Geometry: final body of the model. Coordinates: model frame, mm. Face numbers are marked on the shaded views. A direction names the side the tool comes from. Give positions to 0.01 mm unless a question says otherwise; leave off trailing zeros. Write each loop counter-clockwise with the first axis right and the second up, starting at its lowest first coordinate (ties: lowest second). Pieces come first, ordered by that corner, then holes. Notation, with made-up numbers: (42, 42) -> (50, 42) arc R23 ccw to (50, 54) -> close; hole circle Ø2 at (60, 22.25). An arc over 180 degrees is marked (long way). Answer as a JSON object with one key per item and string values.
from build123d import *

# Parameters (mm, degrees)
F2_R     = 6.2211982037
F3_DEPTH = 19.1516
F4_DEPTH = 55.372
F5_SIZE  = 3.302


# Not quite as in the source:
# - the program builds the solid bodies; features that only make, move or delete a surface that nothing else refers to are left out


with BuildPart() as f1:
    # F0 (on Top) → F1 (revolve)
    with BuildSketch(Plane.XY):
        Polygon((-17.0599853833, 6.2996733477), (-20.4250291926, 4.9693077386), (-13.2254017106, -8.4908647026), (-8.2169655835, -3.2476578449), (-3.9128408491, -8.4126079255), (3.521556964, 4.8910505621), (-2.2694479322, 4.8910505621), (-5.1649496812, 0), (-8.2952223605, 2.6998602059), (-12.2546622766, -1.8907947353), align=None)
    revolve(axis=Axis((-9.930120464, 11.8798027962, 0), (1, 0, 0)))

    # F2 (on Right) → F3 (join)
    with BuildSketch(Plane.YZ):
        with Locations((11.7291258648, 0)):
            Circle(F2_R)
    extrude(amount=-F3_DEPTH)

    # F4 (add): a face of the model
    f4_faces = [f1.faces().sort_by_distance(p)[0] for p in [
        (0, 11.7291258648, 0),
    ]]
    extrude(f4_faces, amount=F4_DEPTH)

    # F5
    f5_edges = [f1.edges().sort_by_distance(p)[0] for p in [
        (55.372, 5.507928, 0),
    ]]
    chamfer(f5_edges, length=F5_SIZE)


solid = f1.part
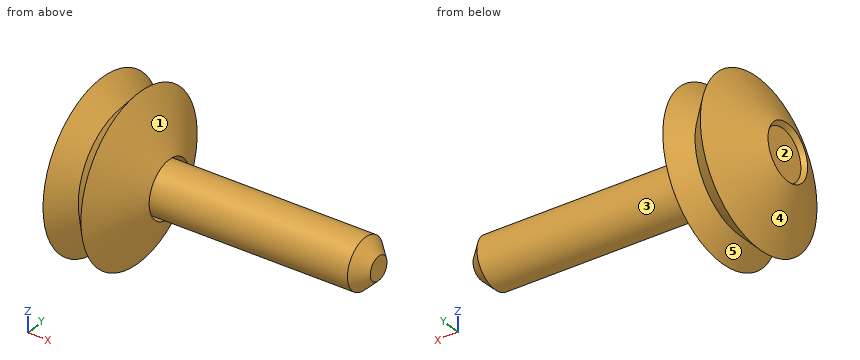
Q1. Set-up query: the marked faces 3, 4 and 5. Return all of +Z, -Z, +X, -X, +Y, -Y with unobstructed straight access to the full face (end or side cutting, diameter ignored); none if empty.
Values:
{"face 3": "+X", "face 4": "-X", "face 5": "none"}
Q2. Material intervals for L1, parallel to Y at x = 1.4, z = 0; L2, parallel to X at y = 1.5, z = -2.5; L3, parallel to Y at x = 2.25, z = 0, sorted ascending. Write a range as from..to.
Values:
{"L1": "1.09..4.89, 5.51..17.95, 18.87..22.67", "L2": "-18.41..-14.07, -9.59..-6.56, -4.45..1.46", "L3": "2.62..4.89, 5.51..17.95, 18.87..21.14"}
Q3. Cut plane B-B (x = 40). Return the cut outline in (y, z), and give its area (3 significant figures).
Values:
{"outline": "circle Ø12.44 at (11.73, 0)", "area": "122 mm²"}
Q4. Cut plane C-C (z = 0). Return the cut outline in (x, y).
Values:
{"outline": "(-20.43, 4.97) -> (-13.23, -8.49) -> (-8.22, -3.25) -> (-3.91, -8.41) -> (3.52, 4.89) -> (-2.27, 4.89) -> (-5.16, 0) -> (-8.3, 2.7) -> (-12.25, -1.89) -> (-16.6, 5.51) -> (52.07, 5.51) -> (55.37, 8.81) -> (55.37, 14.65) -> (52.07, 17.95) -> (-16.77, 17.95) -> (-12.25, 25.65) -> (-8.3, 21.06) -> (-5.16, 23.76) -> (-2.27, 18.87) -> (3.52, 18.87) -> (-3.91, 32.17) -> (-8.22, 27.01) -> (-13.23, 32.25) -> (-20.43, 18.79) -> (-18.3, 17.95) -> (-19.15, 17.95) -> (-19.15, 5.51) -> (-19.06, 5.51) -> close"}
Q5. Cut plane A-A (x = 2.5). Return the cut outline in (y, z).
Values:
{"outline": "circle Ø17.63 at (11.88, 0); circle Ø12.44 at (11.73, 0); hole circle Ø13.98 at (11.88, 0)"}
Q6. First-contact query: P1, Ø13.5, axis at y = 11, z = 2, coming from the -X side (3 decimals); P2, Ø8, axis at x = -2, y = -0.5, coming from the +Z side; P3, Ø3, axis at x = -12, z = -6, coming from the -Y side. Flat tips, straight axial feed; report the tip coordinate or a pass-through.
Values:
{"P1": "x = -20.425", "P2": "z = 18.25", "P3": "y = -7.83"}
Q7. Mould query, pull axis Z, two halves, no side actions, for the marked faces 1 and 2. Classes: pulls with the +Z half, pulls with the -Z half, needs draft (parallel to the pull), parting line crosses it, or undercut.
Values:
{"face 1": "parting line crosses it", "face 2": "undercut"}
